Read the model definition and answer for the solid it produces. Units are mm, in the model's axes. A direction names the side the tool comes from. Coordinates: 2 decimals unless noted, no trailing zeros. Loops run counter-clockwise (first coordinate to the right, second up) from the corner with the lowest first, then second, coordinate; pieces in that order, holes last. Notation, with made-up numbers: M 70.5,-22 L 124.5,-22 A5 ccw 124.5,-18 Z; hole C -9.75,-21 d9. An arc over 180 degrees is marked long. Put each result on its own line as item: value.
from build123d import *

# Parameters (mm, degrees)
F1_DEPTH = 22.7
F2_DEPTH = 50
F3_R     = 5
F5_DEPTH = 50
F4_R     = 5
F6_DEPTH = 50
F7_R     = 2


with BuildPart() as f1:
    # F0 (on Top) → F1 (new body)
    with BuildSketch(Plane.XY):
        Polygon((0, -20), (0, 0), (-20, 0), (-45.358984, -14.641016), (-20, -40), (0, -40), align=None)
        with BuildLine():
            ThreePointArc((-10, -14.641016), (-18.69862, -24.555975), (-29.661282, -17.221643))
            ThreePointArc((-29.661282, -17.221643), (-21.30138, -4.726057), (-10, -14.641016))
        make_face(mode=Mode.SUBTRACT)
        Polygon((-20, 0), (0, 0), (0, 20), (-14.641016, 45.358984), (-40, 20), (-40, 0), align=None)
        with BuildLine():
            ThreePointArc((-4.641016, 20), (-20.731736, 12.068851), (-17.221643, 29.661282))
            ThreePointArc((-17.221643, 29.661282), (-8.550296, 27.931149), (-4.641016, 20))
        make_face(mode=Mode.SUBTRACT)
        with BuildLine():
            ThreePointArc((-4.641016, 20), (-8.550296, 27.931149), (-17.221643, 29.661282))
            ThreePointArc((-17.221643, 29.661282), (-20.731736, 12.068851), (-4.641016, 20))
        make_face()
        with BuildLine():
            ThreePointArc((-10, -14.641016), (-21.30138, -4.726057), (-29.661282, -17.221643))
            ThreePointArc((-29.661282, -17.221643), (-18.69862, -24.555975), (-10, -14.641016))
        make_face()
        Polygon((0, 20), (0, 0), (20, 0), (45.358984, 14.641016), (20, 40), (0, 40), align=None)
        with BuildLine():
            ThreePointArc((30, 14.641016), (10.085041, 13.339636), (29.661282, 17.221643))
            ThreePointArc((29.661282, 17.221643), (29.914959, 15.942396), (30, 14.641016))
        make_face(mode=Mode.SUBTRACT)
        with BuildLine():
            ThreePointArc((24.641016, -20), (6.709867, -13.90928), (17.221643, -29.661282))
            ThreePointArc((17.221643, -29.661282), (22.572166, -26.09072), (24.641016, -20))
        make_face()
        with BuildLine():
            ThreePointArc((30, 14.641016), (29.914959, 15.942396), (29.661282, 17.221643))
            ThreePointArc((29.661282, 17.221643), (10.085041, 13.339636), (30, 14.641016))
        make_face()
        Polygon((20, 0), (0, 0), (0, -20), (14.641016, -45.358984), (40, -20), (40, 0), align=None)
        with BuildLine():
            ThreePointArc((24.641016, -20), (22.572166, -26.09072), (17.221643, -29.661282))
            ThreePointArc((17.221643, -29.661282), (6.709867, -13.90928), (24.641016, -20))
        make_face(mode=Mode.SUBTRACT)
    extrude(amount=F1_DEPTH)

    # F0 (on Top) → F2 (join)
    with BuildSketch(Plane.XY):
        with BuildLine():
            ThreePointArc((-10, -14.641016), (-21.30138, -4.726057), (-29.661282, -17.221643))
            ThreePointArc((-29.661282, -17.221643), (-18.69862, -24.555975), (-10, -14.641016))
        make_face()
        with BuildLine():
            ThreePointArc((-4.641016, 20), (-8.550296, 27.931149), (-17.221643, 29.661282))
            ThreePointArc((-17.221643, 29.661282), (-20.731736, 12.068851), (-4.641016, 20))
        make_face()
        with BuildLine():
            ThreePointArc((30, 14.641016), (29.914959, 15.942396), (29.661282, 17.221643))
            ThreePointArc((29.661282, 17.221643), (10.085041, 13.339636), (30, 14.641016))
        make_face()
        with BuildLine():
            ThreePointArc((24.641016, -20), (6.709867, -13.90928), (17.221643, -29.661282))
            ThreePointArc((17.221643, -29.661282), (22.572166, -26.09072), (24.641016, -20))
        make_face()
    extrude(amount=F2_DEPTH)

    # F3 (on face) → F5 (cut)
    with BuildSketch(Plane.XY.offset(50)):
        with Locations((20, 14.641016)):
            Circle(F3_R)
    extrude(amount=-F5_DEPTH, mode=Mode.SUBTRACT)

    # F3 (on face) + F4 (on face) → F6 (cut)
    with BuildSketch(Plane.XY.offset(50)):
        with Locations((20, 14.641016)):
            Circle(F3_R)
    with BuildSketch(Plane.XY.offset(50)):
        with Locations((-14.641016, 20)):
            Circle(F4_R)
        with Locations((-20, -14.641016)):
            Circle(F4_R)
        with Locations((14.641016, -20)):
            Circle(F4_R)
    extrude(amount=-F6_DEPTH, mode=Mode.SUBTRACT)

    # F7
    f7_edges = [f1.edges().sort_by_distance(p)[0] for p in [
        (-10.338718, -12.06039, 50),
        (12.06039, -10.338718, 50),
        (10, 14.641016, 50),
        (-24.641016, 20, 50),
    ]]
    fillet(f7_edges, radius=F7_R)


solid = f1.part
1) Find section A-A, the plane z = 11.5. Write down the section's boundary in (x, y).
Answer list:
outline: M -45.36,-14.64 L -20,-40 L 0,-40 L 0,-20 L 14.64,-45.36 L 40,-20 L 40,0 L 20,0 L 45.36,14.64 L 20,40 L 0,40 L 0,20 L -14.64,45.36 L -40,20 L -40,0 L -20,0 Z; hole C -20,-14.64 d10; hole C -14.64,20 d10; hole C 14.64,-20 d10; hole C 20,14.64 d10
2) Find section B-B, the plane x = 32. Write down the section's boundary in (y, z), plus the area to 3 significant figures.
Answer list:
outline: M -28,0 L 0,0 L 0,22.7 L -28,22.7 Z; M 6.93,0 L 28,0 L 28,22.7 L 6.93,22.7 Z
area: 1,110 mm^2
3) Find section C-C, the plane y = 3. Write down the section's boundary in (x, z).
Answer list:
outline: M -40,0 L 25.2,0 L 25.2,22.7 L -40,22.7 Z
4) Determine the mould class of faces 1 (the flat face through (33, 27, 11)), 2 (the flat face through (-24, -18, 50)), 3 (the flat face through (-30, 0, 11)), 4 (the cylindrical face through (-21.084, -19.522, 25.35)) for opening direction Y: released by +Y, released by -Y, zero draft, split by the parting line, or undercut.
Answer list:
face 1: released by +Y
face 2: zero draft
face 3: undercut
face 4: undercut
5) Which of the six approach directions +Z, -Z, +X, -X, +Y, -Y give full straight-line access (tool end or side, diameter ignored) to faces 5 (the flat face through (-10, -40, 11)), 6 (the flat face through (32.502, 7.218, 11.191)), 7 (the flat face through (-40, 10, 11)), 8 (the flat face through (7.218, -32.502, 11.191))?
Answer list:
face 5: +Z, -Z, -X, -Y
face 6: +Z, -Z, +X
face 7: +Z, -Z, -X, +Y
face 8: +Z, -Z, -Y
6) Given pin 1 Ø3 at (x, z) = (-6, 20.5) entering from -Y; pin 2 Ø6 at (x, z) = (-34, 12) entering from -Y; pin 3 Ø6 at (x, y) = (-6, 28) entering from +Z, each flat-ended and moving along its own axis, determine where each tip first touches the part or whether it passes through.
Answer list:
pin 1: stops at y = -40
pin 2: stops at y = -29
pin 3: stops at z = 49.84
7) Straight lines are drawn through the part: line 1 (Y direction, x = 22, z = 44); line 2 (X direction, y = -18, z = 25); line 3 (X direction, y = 16, z = 33). For each, find the intervals that lie inside material, in ascending order. Write a range as [from, to].
Answer list:
line 1: y = [-26.77, -13.23], [4.84, 10.06], [19.22, 24.44]
line 2: x = [-29.42, -23.7], [-16.3, -10.58], [4.84, 10.06], [19.22, 24.44]
line 3: x = [-23.81, -17.64], [-11.64, -5.48], [10.09, 15.19], [24.81, 29.91]
